For this review, take the finished solid that the model builds, in its own axes (mm). Coordinates: 2 decimals unless noted, no trailing zeros. Write each loop counter-clockwise with the first axis right and the second up, starting at its lowest first coordinate (ties: lowest second). Pieces come first, ordered by that corner, then holes. Notation, with made-up numbers: (35.25, -12) -> (65.25, -12) arc R38 cw to (65.25, 26) -> close; hole circle Ø7 at (25.5, 59). An arc over 180 degrees is marked (long way). Put each result on its own line as item: value. Start each with the question number.
Item 1: Consider section B-B on z = 0. Give the boundary of the cut face in (x, y), and give its area (3 significant figures).
Item 2: Consider section D-D on y = 0.4. Give the number of separate pieces and of enclosed holes in the cut face, and give its area (3 significant figures).
Item 3: Consider section A-A on x = 150. Give the boundary of the cut face in (y, z).
Item 4: To check wall thickness, follow L1, parallel to X at y = 0.6, z = 0; L2, parallel to X at y = 1.5, z = 9; L3, parallel to Z at x = 31.5, y = 0.65. State the ranges of each line that lie inside material, in increasing order.
Item 5: Insertion check: P1, Ø1, axis at x = 227.5, y = 1.5, coming from the -Z side; P2, Ø6, axis at x = 238, z = 23, coming from the -Y side; P3, Ø1, axis at y = 1, z = 31.5, coming from the -X side; P4, Ø0.6, axis at y = 0.5, z = 24, coming from the -X side. Each pin has a flat end and moves straight along its axis. Give the tip position at first contact, or say it passes through.
Item 6: Consider section C-C on x = 200. Give the boundary of the cut face in (y, z), and give its area (3 significant figures).
```python
from build123d import *

# Parameters (mm, degrees)
SKETCH_1_R      = 5
SKETCH_1_W      = 2
SKETCH_1_H      = 30
SKETCH_1_W_2    = 105
SKETCH_1_H_2    = 50
SKETCH_1_R_2    = 3
SKETCH_1_H_3    = 7.4
SKETCH_1_W_3    = 40
SKETCH_1_H_4    = 2
SKETCH_1_W_4    = 70
EXTRUDE_1_DEPTH = 2


with BuildPart() as part:
    # 草图1 → 凸台-拉伸1 (new body)
    # profile 1 of 5: a face of its own
    with BuildSketch(Plane(origin=(0, 0, 0), x_dir=(1, 0, 0), z_dir=(0, 1, 0))):
        Polygon((-2, 20), (-2, -20), (0, -20), (0, -30), (50, -30), (90, -30), (135, -30), (205, -30), (275, -30), (275, 30), (205, 30), (135, 30), (90, 30), (50, 30), (0, 30), (0, 20), align=None)
        with Locations(Location((150, -15, 0), (0, 0, 270))):
            Circle(SKETCH_1_R, mode=Mode.SUBTRACT)
        with Locations((9, 0)):
            Rectangle(SKETCH_1_W, SKETCH_1_H, mode=Mode.SUBTRACT)
        with Locations((72.5, 0)):
            Rectangle(SKETCH_1_W_2, SKETCH_1_H_2, mode=Mode.SUBTRACT)
        with Locations((136, 0)):
            Rectangle(SKETCH_1_W, SKETCH_1_H, mode=Mode.SUBTRACT)
        with Locations(Location((200, 0, 0), (0, 0, 270))):
            Circle(SKETCH_1_R_2, mode=Mode.SUBTRACT)
        with Locations((233.7, 0)):
            Rectangle(SKETCH_1_W, SKETCH_1_H_3, mode=Mode.SUBTRACT)
    # profile 2 of 5: a face of its own
    with BuildSketch(Plane(origin=(0, 0, 0), x_dir=(1, 0, 0), z_dir=(0, 1, 0))):
        with Locations((70, 31)):
            Rectangle(SKETCH_1_W_3, SKETCH_1_H_4)
    # profile 3 of 5: a face of its own
    with BuildSketch(Plane(origin=(0, 0, 0), x_dir=(1, 0, 0), z_dir=(0, 1, 0))):
        with Locations((170, 31)):
            Rectangle(SKETCH_1_W_4, SKETCH_1_H_4)
    # profile 4 of 5: a face of its own
    with BuildSketch(Plane(origin=(0, 0, 0), x_dir=(1, 0, 0), z_dir=(0, 1, 0))):
        with Locations((70, -31)):
            Rectangle(SKETCH_1_W_3, SKETCH_1_H_4)
    # profile 5 of 5: a face of its own
    with BuildSketch(Plane(origin=(0, 0, 0), x_dir=(1, 0, 0), z_dir=(0, 1, 0))):
        with Locations((170, -31)):
            Rectangle(SKETCH_1_W_4, SKETCH_1_H_4)
    extrude(amount=EXTRUDE_1_DEPTH)


solid = part.part
```
Return value:
1. outline: (-2, 0) -> (8, 0) -> (8, 2) -> (-2, 2) -> close; (10, 0) -> (20, 0) -> (20, 2) -> (10, 2) -> close; (125, 0) -> (135, 0) -> (135, 2) -> (125, 2) -> close; (137, 0) -> (197, 0) -> (197, 2) -> (137, 2) -> close; (203, 0) -> (232.7, 0) -> (232.7, 2) -> (203, 2) -> close; (234.7, 0) -> (275, 0) -> (275, 2) -> (234.7, 2) -> close
1. area: 320 mm^2
2. separate pieces: 1
2. enclosed holes: 6
2. area: 11,500 mm^2
3. outline: (0, -32) -> (2, -32) -> (2, 10) -> (0, 10) -> close; (0, 20) -> (2, 20) -> (2, 32) -> (0, 32) -> close
4. L1: -2 to 8, 10 to 20, 125 to 135, 137 to 197, 203 to 232.7, 234.7 to 275
4. L2: -2 to 8, 10 to 20, 125 to 135, 137 to 275
4. L3: -30 to -25, 25 to 30
5. P1: z = -30
5. P2: y = 0
5. P3: x = 50
5. P4: x = 0
6. outline: (0, -32) -> (2, -32) -> (2, -3) -> (0, -3) -> close; (0, 3) -> (2, 3) -> (2, 32) -> (0, 32) -> close
6. area: 116 mm^2
